Answer from the drawing. Dimensions are ordinates in mm from the lowest x, y and z of the part. Round coordinates to 2 decimals unless told otherwise and drop trailing zeros. Write each loop counter-clockwise with the first axis right and the second up, starting at its lowest first coordinate (ties: lowest second). Pieces come first, ordered by that corner, then holes. Notation, with made-up numbers: (20, 7) - (65, 7) arc R20 cw to (65, 16) - close; hole circle Ø2 at (42, 54.5). An arc over 180 degrees is marked (long way). Answer in a Markdown table with one row per item.
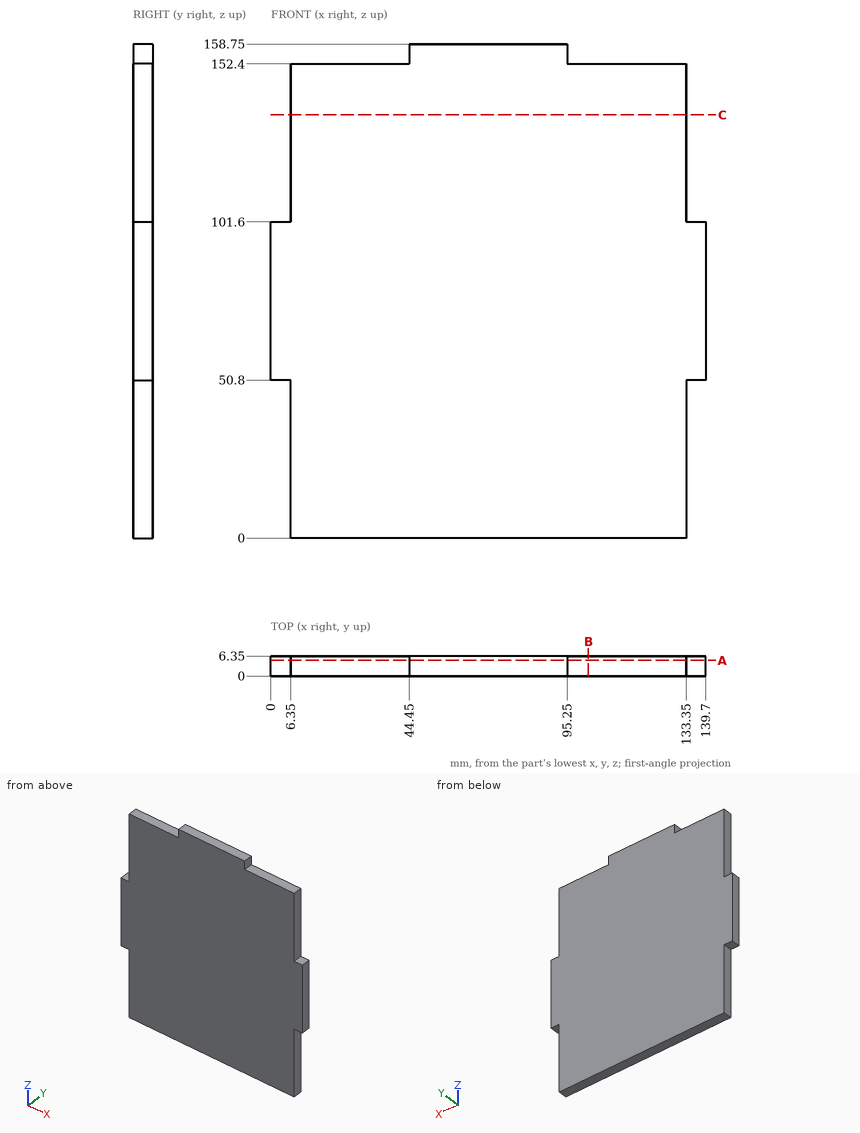
(1) Section B-B (x = 102) is taken. Give the vertices of the cut face in (y, z), and give its area (3 significant figures).
Checked values:
| item | result |
|---|---|
| outline | (0, 0) - (6.35, 0) - (6.35, 152.4) - (0, 152.4) - close |
| area | 968 mm2 |
(2) Find the intervals of material crossed by line 1 (X direction, y = 4.75, z = 139.5); line 2 (Z direction, x = 133.5, y = 5.5); line 3 (Z direction, x = 131, y = 6), in increasing order.
Checked values:
| item | result |
|---|---|
| line 1 | x = 6.35 to 133.35 |
| line 2 | z = 50.8 to 101.6 |
| line 3 | z = 0 to 152.4 |
(3) Section C-C (z = 136) is taken. Give the vertices of the cut face in (x, y).
Checked values:
| item | result |
|---|---|
| outline | (6.35, 0) - (133.35, 0) - (133.35, 6.35) - (6.35, 6.35) - close |
(4) Flat-ended cylindrical pins translate along their axes: pin 1 (1.9 mm diameter, centred on x = 137.5, y = 3, fed in from -Z); pin 2 (3 mm diameter, centred on y = 2, z = 32.5, fed in from -X); pin 3 (3 mm diameter, centred on x = 119.5, y = 2, fed in from +Z). Find the tip coordinate at first contact, or state that the pin passes through.
Checked values:
| item | result |
|---|---|
| pin 1 | stops at z = 50.8 |
| pin 2 | stops at x = 6.35 |
| pin 3 | stops at z = 152.4 |
(5) Section A-A (y = 5) is taken. Give the vertices of the cut face in (x, z), and give its area (3 significant figures).
Checked values:
| item | result |
|---|---|
| outline | (0, 50.8) - (6.35, 50.8) - (6.35, 0) - (133.35, 0) - (133.35, 50.8) - (139.7, 50.8) - (139.7, 101.6) - (133.35, 101.6) - (133.35, 152.4) - (95.25, 152.4) - (95.25, 158.75) - (44.45, 158.75) - (44.45, 152.4) - (6.35, 152.4) - (6.35, 101.6) - (0, 101.6) - close |
| area | 20,300 mm2 |
